The listing builds one solid part. Answer for the finished solid, in the listing's coordinates (mm). Face numbers are marked on the shaded views. A direction names the side the tool comes from. Round coordinates to 2 decimals unless told otherwise and drop trailing zeros. Write each loop counter-clockwise with the first axis right and the second up, starting at its lowest first coordinate (ties: lowest second). Pieces come first, ordered by that corner, then holes.
(1) A cutting plane is placed at A-A, the plane y = -5.25. Give the vertices of the cut face in (x, z).
(2) Find the intervals of material crossed by probe 1 along Z at (x, y) = (6.75, 0); probe 2 along Y at (x, z) = (-0.5, 92), in increasing order.
(3) For the marked faces 5 and 6, determine the directions among +Z, -Z, +X, -X, +Y, -Y from which every point of the face is accessible in a straight line to the end or side of a thin tool.
(4) A cutting plane is placed at B-B, the plane z = 26.5. Give the vertices of the cut face in (x, y), and give its area (3 significant figures).
(5) The mould has two halves that part along X. Classify the marked faces 1, 2, 3 and 4: +X half, -X half, draft (parallel to the pull), parting line (faces both ways), or undercut.
(6) This flat-tipped pin is pushed along its axis until it touches: pin 1 Ø3.5 at (x, z) = (0, 69.25) entering from -Y. Where does it stop, or does it pass through?
(7) A cutting plane is placed at D-D, the plane y = 0. Give the number of separate pieces and of enclosed holes in the cut face, and give its area (3 significant figures).
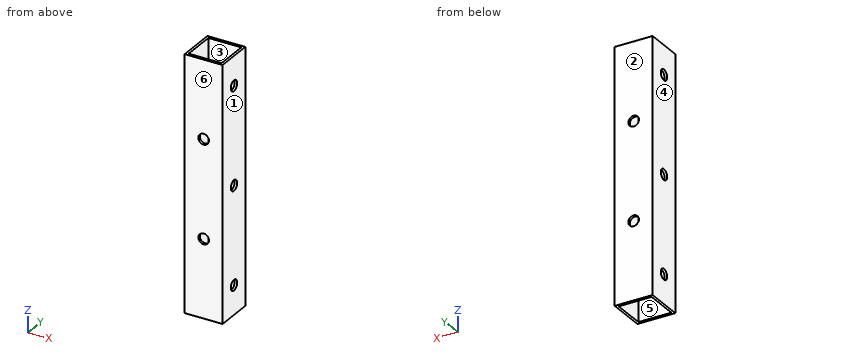
from build123d import *

# Parameters (mm, degrees)
SKETCH_1_W          = 15
SKETCH_1_H          = 15
SKETCH_1_W_2        = 13
SKETCH_1_H_2        = 13
EXTRUDE_1_DEPTH     = 100
SKETCH_2_R          = 2.1
CUT_EXTRUDE_1_DEPTH = 366
SKETCH_3_R          = 2.1
CUT_EXTRUDE_2_DEPTH = 55


with BuildPart() as part:
    # 草图1 → 凸台-拉伸1 (new body)
    with BuildSketch(Plane.XY):
        Rectangle(SKETCH_1_W, SKETCH_1_H)
        Rectangle(SKETCH_1_W_2, SKETCH_1_H_2, mode=Mode.SUBTRACT)
    extrude(amount=EXTRUDE_1_DEPTH)

    # 草图2 → 切除-拉伸1 (cut)
    with BuildSketch(Plane(origin=(7.5, 0, 0), x_dir=(0, 0, -1), z_dir=(1, 0, 0))):
        with Locations(Location((-50, 0, 0), (0, 0, 90))):
            Circle(SKETCH_2_R)
        with Locations(Location((-88.5, 0, 0), (0, 0, 90))):
            Circle(SKETCH_2_R)
        with Locations(Location((-11.5, 0, 0), (0, 0, 90))):
            Circle(SKETCH_2_R)
    extrude(amount=-CUT_EXTRUDE_1_DEPTH, mode=Mode.SUBTRACT)

    # 草图3 → 切除-拉伸2 (cut)
    with BuildSketch(Plane(origin=(0, 7.5, 0), x_dir=(1, 0, 0), z_dir=(0, 1, 0))):
        with Locations(Location((0, -30.75, 0), (0, 0, 270))):
            Circle(SKETCH_3_R)
        with Locations(Location((0, -69.25, 0), (0, 0, 270))):
            Circle(SKETCH_3_R)
    extrude(amount=-CUT_EXTRUDE_2_DEPTH, mode=Mode.SUBTRACT)


solid = part.part
Solutions:
1. outline: (-7.5, 0) - (-6.5, 0) - (-6.5, 100) - (-7.5, 100) - close; (6.5, 0) - (7.5, 0) - (7.5, 100) - (6.5, 100) - close
2. probe 1: z = 0 to 9.4, 13.6 to 47.9, 52.1 to 86.4, 90.6 to 100
2. probe 2: y = -7.5 to -6.5, 6.5 to 7.5
3. face 5: +Z, -Z
3. face 6: +Z, -Z, +X, -X, -Y
4. outline: (-7.5, -7.5) - (7.5, -7.5) - (7.5, 7.5) - (-7.5, 7.5) - close; hole (-6.5, -6.5) - (6.5, -6.5) - (6.5, 6.5) - (-6.5, 6.5) - close
4. area: 56.0 mm2
5. face 1: +X half
5. face 2: draft
5. face 3: undercut
5. face 4: -X half
6. pin 1: passes through
7. separate pieces: 8
7. enclosed holes: 0
7. area: 175 mm2
